```python
from build123d import *

# Parameters (mm, degrees)
FILLET2_R = 2


with BuildPart() as part:
    # Sketch1 → Revolve1 (revolve)
    with BuildSketch(Plane.XY):
        Polygon((-14.412217993, 18.021334137), (-14.412217993, 17.213777129), (-11.987191568, 10.920560913), (-11.987191568, 7.870061872), (-12.453293915, 7.870061872), (-12.453293915, 6.766705429), (-11.987191568, 6.766705429), (13.120112204, 6.766705429), (13.74017448, 6.766705429), (13.74017448, 7.870061872), (13.120112204, 7.870061872), (13.120112204, 10.920560913), (15.416727783, 17.213777129), (15.416727783, 18.021334137), align=None)
    revolve(axis=Axis((76.351551313, 0, 0), (-1, 0, 0)))

    # Fillet2
    fillet2_edges = [part.edges().sort_by_distance(p)[0] for p in [
        (15.416727783, -17.213777129, 0),
        (13.120112204, -10.920560913, 0),
        (-11.987191568, -10.920560913, 0),
        (-14.412217993, -17.213777129, 0),
    ]]
    fillet(fillet2_edges, radius=FILLET2_R)


solid = part.part
```
The listing builds one solid part. Answer for the finished solid, in the listing's coordinates (mm). A direction names the side the tool comes from. Round coordinates to 2 decimals unless told otherwise and drop trailing zeros. Order: outer loops, then holes, each group sorted by start corner. A loop starts at its lowest first (then second) coordinate and runs counter-clockwise, first axis right, second up. Notation, with made-up numbers: (12.25, 23) - (67.25, 23) arc R29 ccw to (67.25, 48) - close; hole circle Ø11 at (87.25, 24). An arc over 180 degrees is marked (long way). Put each result on its own line as item: value. Start each with the question number.
(1) Given P1, Ø4, axis at y = 3.5, z = 7, coming from the -X side; P2, Ø3, axis at x = 9, z = -8.5, coming from the -Y side; P3, Ø6, axis at y = -5, z = 10, coming from the -X side, each flat-ended and moving along its own axis, determine where each tip first touches the part or whether it passes through.
(2) For faces 4 (the cylindrical face through (13.426, 7.507, -2.364)), 5 (the flat face through (-14.412, 15.9, 7.9)), 6 (the flat face through (-12.453, -4, -6)), determine the directions among +Z, -Z, +X, -X, +Y, -Y from which every point of the face is accessible in a straight line to the end or side of a thin tool.
(3) Straight lines are drawn through the part: probe 1 along Y at (x, z) = (-1.5, 0); probe 2 along X at (y, z) = (-10, 3). For each, find the intervals that lie inside material, in ascending order. Write a range as from..to.
(4) Find section C-C (x = 0). Give the vertices of the cut face in (y, z), plus the area to 3 significant figures.
(5) Determine the mould class of faces 1 (the flat face through (13.74, 4, -6)), 2 (the flat face through (15.417, -17.3, 3.9)), 3 (the cylindrical face through (0.29, -13.28, -12.18)) for opening direction Y: released by +Y, released by -Y, zero draft, split by the parting line, or undercut.
Reply:
1. P1: x = -12.45
1. P2: y = -16.61
1. P3: x = -13.24
2. face 4: +X
2. face 5: +Z, -Z, -X, +Y, -Y
2. face 6: -X
3. probe 1: -18.02..-6.77, 6.77..18.02
3. probe 2: -11.99..13.12
4. outline: circle Ø36.04 at (0, 0); hole circle Ø13.53 at (0, 0)
4. area: 876 mm^2
5. face 1: undercut
5. face 2: zero draft
5. face 3: split by the parting line
